Check sheet for the drawn part. Datum: minimum x, y, z corner. Units: mm. Coordinates: 2 decimals unless noted, no trailing zeros. Loops run counter-clockwise (first coordinate to the right, second up) from the corner with the lowest first, then second, coordinate; pieces in that order, holes last. Notation, with made-up numbers: M 6.25,30 L 11.25,30 A15 cw 11.25,59 Z; hole C 22,-25 d6. An arc over 180 degrees is marked long. Answer in a Markdown table with one row per item. Add a question column.
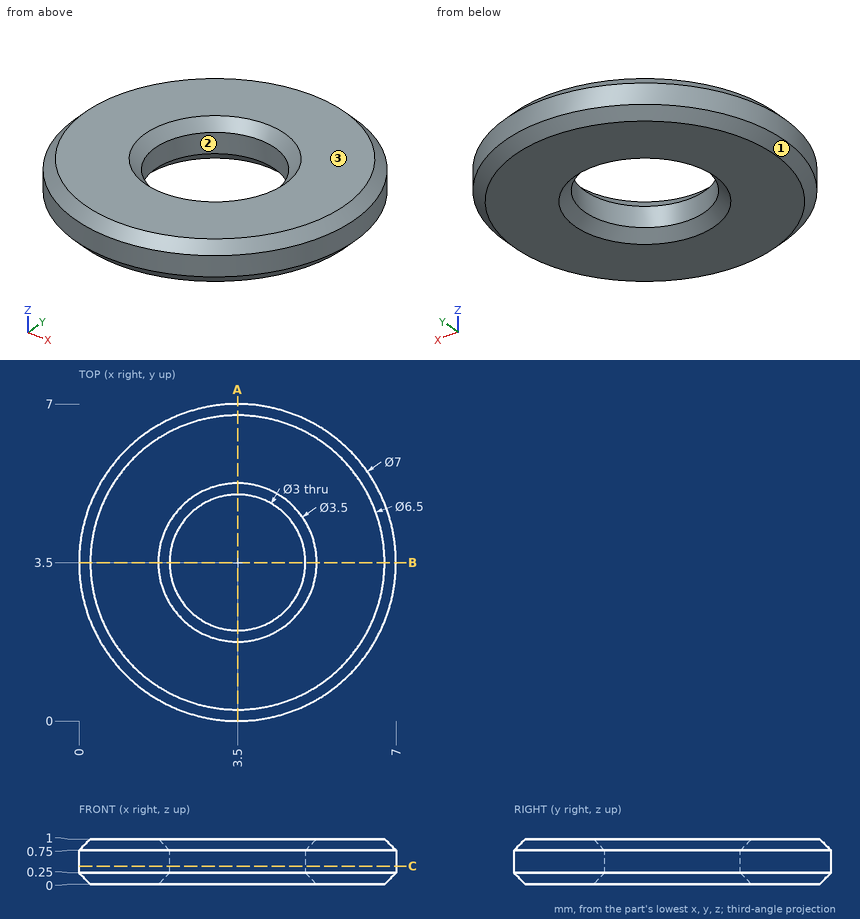
Q1. Cross-section at C-C (z = 0.4). Record the cut outline in (x, y), plus the area to 3 significant figures.
Q2. Thickness scan on L1, parallel to Y at x = 3.5, z = 0.4; L2, parallel to Y at x = 4, z = 0.55; L3, parallel to X at y = 4.75, z = 0.15. Record the ranges inside material, lowest first.
Q3. Go/stop test with a flat-tipped pin: pin 1 (1.5 mm diameter, centred on x = 4, y = 3, fed in from -Z). Record where the tip stops, or that it passes through.
Q4. Cross-section at A-A (x = 3.5). Record the cut outline in (y, z), plus the area to 3 significant figures.
Q5. Mould release check, pull along Y, two halves, no side actions. Record for the marked faces 1, 2 and 3: released by +Y, released by -Y, zero draft, split by the parting line, or undercut.
Answer key:
| question | item | result |
|---|---|---|
| 1 | outline | C 3.5,3.5 d7; hole C 3.5,3.5 d3 |
| 1 | area | 31.4 mm^2 |
| 2 | L1 | 0 to 2, 5 to 7 |
| 2 | L2 | 0.04 to 2.09, 4.91 to 6.96 |
| 2 | L3 | 0.34 to 2.5, 4.5 to 6.66 |
| 3 | pin 1 | through |
| 4 | outline | M 0,0.25 L 0.25,0 L 1.75,0 L 2,0.25 L 2,0.75 L 1.75,1 L 0.25,1 L 0,0.75 Z; M 5,0.25 L 5.25,0 L 6.75,0 L 7,0.25 L 7,0.75 L 6.75,1 L 5.25,1 L 5,0.75 Z |
| 4 | area | 3.75 mm^2 |
| 5 | face 1 | split by the parting line |
| 5 | face 2 | undercut |
| 5 | face 3 | zero draft |
